```python
from build123d import *

# Parameters (mm, degrees)
ESQUISSE1_R             = 55
ESQUISSE1_R_2           = 35
BOSS_EXTRU_1_DEPTH      = 20
CONG_6_R                = 1
ESQUISSE3_R             = 49.95
ESQUISSE3_R_2           = 41.45
ENL_V_MAT_EXTRU_1_DEPTH = 4


with BuildPart() as part:
    # Esquisse1 → Boss.-Extru.1 (new body)
    with BuildSketch(Plane.XY):
        Circle(ESQUISSE1_R)
        Circle(ESQUISSE1_R_2, mode=Mode.SUBTRACT)
    extrude(amount=BOSS_EXTRU_1_DEPTH)

    # Congé6
    cong_6_edges = [part.edges().sort_by_distance(p)[0] for p in [
        (-55, 0, 0),
        (-55, 0, 20),
        (-35, 0, 0),
        (-35, 0, 20),
    ]]
    fillet(cong_6_edges, radius=CONG_6_R)

    # Esquisse3 → Enlèv. mat.-Extru.1 (cut)
    with BuildSketch(Plane(origin=(0, 0, 0), x_dir=(-1, 0, 0), z_dir=(0, 0, -1))):
        Circle(ESQUISSE3_R)
        Circle(ESQUISSE3_R_2, mode=Mode.SUBTRACT)
    extrude(amount=-ENL_V_MAT_EXTRU_1_DEPTH, mode=Mode.SUBTRACT)


solid = part.part
```
Can you work these out from the model? Positions are in its coordinate system, mm. A direction names the side the tool comes from. Give positions to 0.01 mm unless a question says otherwise; leave off trailing zeros. Loops run counter-clockwise (first coordinate to the right, second up) from the corner with the lowest first, then second, coordinate; pieces in that order, holes last. Notation, with made-up numbers: M 50.5,31.25 L 60.5,31.25 A20 ccw 60.5,61.25 Z; hole C -39.75,41.5 d5. An arc over 180 degrees is marked long. Answer in a Markdown table with one row per item.
1. Suppose I cut it at A-A on x = 0. Write out the boundary of the cut face in (y, z), plus the area to 3 significant figures.
Taken from the geometry:
| item | result |
|---|---|
| outline | M -55,1 A1 ccw -54,0 L -49.95,0 L -49.95,4 L -41.45,4 L -41.45,0 L -36,0 A1 ccw -35,1 L -35,19 A1 ccw -36,20 L -54,20 A1 ccw -55,19 Z; M 35,1 A1 ccw 36,0 L 41.45,0 L 41.45,4 L 49.95,4 L 49.95,0 L 54,0 A1 ccw 55,1 L 55,19 A1 ccw 54,20 L 36,20 A1 ccw 35,19 Z |
| area | 730 mm² |
2. For pin 1 Ø1.5 at (x, z) = (8.5, 16) entering from -Y; pin 2 Ø3 at (y, z) = (-5, 9.5) entering from +X; pin 3 Ø6 at (x, z) = (1.5, 2) entering from -Y; pin 4 Ø6 at (y, z) = (-0.5, 14.5) entering from +X, each with a flat end and sliding along its axis, tell me the tip position at first contact or that it passes through.
Taken from the geometry:
| item | result |
|---|---|
| pin 1 | stops at y = -54.45 |
| pin 2 | stops at x = 54.89 |
| pin 3 | stops at y = -55 |
| pin 4 | stops at x = 55 |
3. Which directions (+Z, -Z, +X, -X, +Y, -Y) give clear straight access to the entire face, cutting with the end or side of a thin tool? Please do faces 1 (the cylindrical face through (10.83, -48.76, 1.97)), 2 (the flat face through (35, -11, 20)).
Taken from the geometry:
| item | result |
|---|---|
| face 1 | -Z |
| face 2 | +Z, +X, -X, +Y, -Y |
4. If I drill on line 1 along Y through (x, z) = (0, 1.3); line 2 along Y through (x, z) = (0, 10); line 3 along Z through (x, y) = (30.5, -38), over which ranges is the centre line in solid material (lowest first)?
Taken from the geometry:
| item | result |
|---|---|
| line 1 | y = -55 to -49.95, -41.45 to -35, 35 to 41.45, 49.95 to 55 |
| line 2 | y = -55 to -35, 35 to 55 |
| line 3 | z = 4 to 20 |
5. Thinking about a two-plate mould opening in X: for faces 3 (the cylindrical face through (32.893, -25.222, 1.972)), 4 (the flat face through (48, -16, 0)), 5 (the cylindrical face through (-11.923, -53.692, 9.874)), which applies, released by +X, released by -X, zero draft, split by the parting line, or undercut?
Taken from the geometry:
| item | result |
|---|---|
| face 3 | undercut |
| face 4 | zero draft |
| face 5 | split by the parting line |
6. Suppose I cut it at C-C on z = 15.25. Write out the boundary of the cut face in (x, y).
Taken from the geometry:
| item | result |
|---|---|
| outline | C 0,0 d110; hole C 0,0 d70 |
